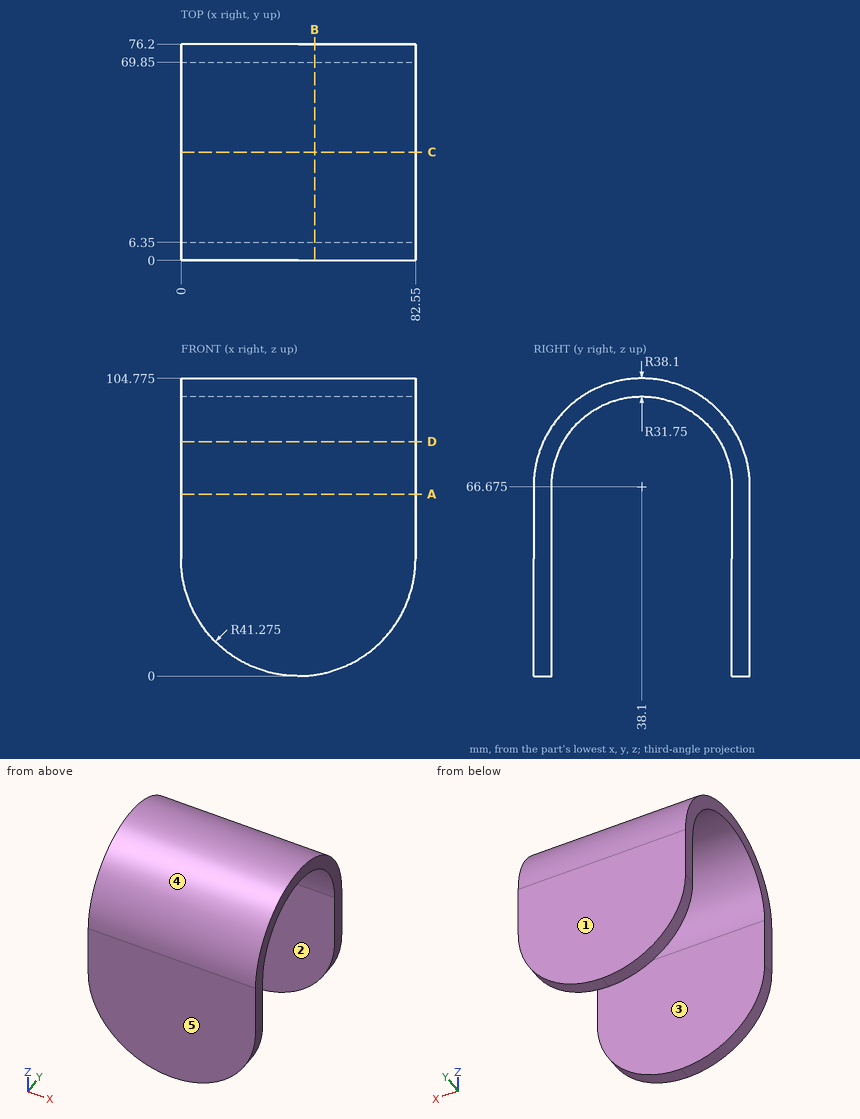
The drawing under review shows one solid part. Ordinate dimensions are in mm from its lowest x, y, z. A direction names the side the tool comes from. Coordinates: 2 decimals unless noted, no trailing zeros. Write each loop counter-clockwise with the first axis right and the second up, starting at its lowest first coordinate (ties: lowest second). Pieces come first, ordered by that corner, then holes. Notation, with made-up numbers: M 68,14 L 86,14 A11 cw 86,28 Z; hole C 77,61 d6. An arc over 180 degrees is marked long. Put each result on its own line as item: value.
1) Wall thickness on probe 1 along Y at (x, z) = (63, 26.5); probe 2 along Y at (x, z) = (17, 79.5); probe 3 along Z at (x, y) = (58.5, 64): over which ranges is each line inside the solid? List them lowest first. Write a range as [from, to].
Computed:
probe 1: y = [0, 6.35], [69.85, 76.2]
probe 2: y = [2.22, 9.06], [67.14, 73.98]
probe 3: z = [85.04, 94.62]
2) Add section C-C on y = 38.1. Give the boundary of the cut face in (x, z) (3 decimals).
Computed:
outline: M 0,98.425 L 82.55,98.425 L 82.55,104.775 L 0,104.775 Z
3) Add section B-B on x = 47. Give the boundary of the cut face in (y, z) (3 decimals), then the cut area to 3 significant figures.
Computed:
outline: M 0,0.399 L 6.35,0.399 L 6.35,66.675 A31.75 cw 69.85,66.675 L 69.85,0.399 L 76.2,0.399 L 76.2,66.675 A38.1 ccw 0,66.675 Z
area: 1,540 mm2
4) Add section A-A on z = 64. Give the boundary of the cut face in (x, y).
Computed:
outline: M 0,0 L 82.55,0 L 82.55,6.35 L 0,6.35 Z; M 0,69.85 L 82.55,69.85 L 82.55,76.2 L 0,76.2 Z
5) Add section D-D on z = 82.5. Give the boundary of the cut face in (x, y), then the cut area to 3 significant figures.
Computed:
outline: M 0,3.44 L 82.55,3.44 L 82.55,10.57 L 0,10.57 Z; M 0,65.63 L 82.55,65.63 L 82.55,72.76 L 0,72.76 Z
area: 1,180 mm2
6) For the marked faces 1 and 2, list the 3-axis set-ups (+Z, -Z, +X, -X, +Y, -Y) from which the entire face can be reached by the end or side of a thin tool; tool diameter is ignored.
Computed:
face 1: +Z, -Z, +X, -X, +Y
face 2: -Z, +X, -X
7) Draft analysis for pull direction Y (two halves, no side actions). For the marked faces 3, 4 and 5, state which applies: released by +Y, released by -Y, zero draft, split by the parting line, or undercut.
Computed:
face 3: undercut
face 4: split by the parting line
face 5: released by -Y
8) Clearance check with flat-ended pins moving along their axes: pin 1 Ø3 at (x, y) = (54.5, 53.5) entering from +Z; pin 2 Ø4 at (x, z) = (18.5, 58) entering from -Y; pin 3 Ø8 at (x, y) = (21.5, 24) entering from -Z; pin 4 Ø3 at (x, z) = (14.5, 86) entering from -Y. State where each tip first meets the part, or that it passes through.
Computed:
pin 1: stops at z = 102.15
pin 2: stops at y = 0
pin 3: stops at z = 92.76
pin 4: stops at y = 4.43
